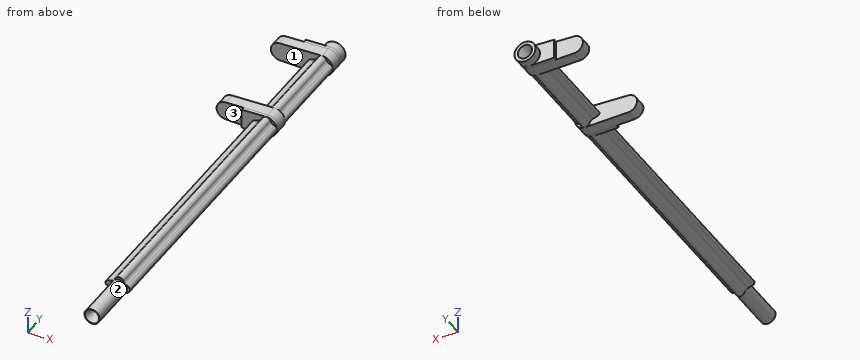
from build123d import *

# Parameters (mm, degrees)
SALIENTE_EXTRUIR2_DEPTH = 223
SALIENTE_EXTRUIR3_DEPTH = 7
SALIENTE_EXTRUIR4_DEPTH = 2
CROQUIS7_R              = 6.250085867
SALIENTE_EXTRUIR5_DEPTH = 5
CROQUIS8_R              = 4.25
CROQUIS9_R              = 1
CROQUIS10_R             = 4.57471759
SALIENTE_EXTRUIR6_DEPTH = 30


with BuildPart() as part:
    # Croquis1 → Saliente-Extruir2 (new body)
    with BuildSketch(Plane(origin=(0, 0, 0), x_dir=(1, 0, 0), z_dir=(0, 1, 0))):
        with BuildLine():
            Line((-14.479902674, 6.344412478), (-17.285197352, 5.373069954))
            ThreePointArc((-17.285197352, 5.373069954), (-18.294405629, 3.955634423), (-17.285197352, 2.538198891))
            Line((-17.285197352, 2.538198891), (-14.479902674, 1.566856368))
            ThreePointArc((-14.479902674, 1.566856368), (-13.134902489, 0.727156406), (-12.288428502, -0.61359089))
            ThreePointArc((-12.288428502, -0.61359089), (-9.893736846, -2.309516044), (-7.499045189, -0.61359089))
            ThreePointArc((-7.499045189, -0.61359089), (-6.663048477, 0.716688354), (-5.33552109, 1.557048043))
            ThreePointArc((-5.33552109, 1.557048043), (-3.642743095, 3.955634423), (-5.33552109, 6.354220802))
            ThreePointArc((-5.33552109, 6.354220802), (-6.654198374, 7.185732469), (-7.490653659, 8.501279498))
            ThreePointArc((-7.490653659, 8.501279498), (-9.893736846, 10.190483956), (-12.296820032, 8.501279498))
            ThreePointArc((-12.296820032, 8.501279498), (-13.143789356, 7.175301343), (-14.479902674, 6.344412478))
        make_face()
    extrude(amount=SALIENTE_EXTRUIR2_DEPTH)

    # Croquis5 → Saliente-Extruir3 (add)
    with BuildSketch(Plane(origin=(0, 223, 0), x_dir=(1, 0, 0), z_dir=(0, 1, 0))):
        with BuildLine():
            Line((-10.079327793, 10.188632247), (-35.332864115, 9.438053784))
            ThreePointArc((-35.332864115, 9.438053784), (-40.669466825, 3.940481472), (-35.332864115, -1.55709084))
            Line((-35.332864115, -1.55709084), (-10.079327793, -2.307669303))
            ThreePointArc((-10.079327793, -2.307669303), (-3.64271211, 3.940481472), (-10.079327793, 10.188632247))
        make_face()
    saliente_extruir3 = extrude(amount=SALIENTE_EXTRUIR3_DEPTH)

    # Croquis6 → Saliente-Extruir4 (add)
    with BuildSketch(Plane(origin=(0, 230, 0), x_dir=(1, 0, 0), z_dir=(0, 1, 0))):
        with BuildLine():
            Line((-24.6694675, 9.754988242), (-10.105220694, 10.18780896))
            ThreePointArc((-10.105220694, 10.18780896), (-3.64271211, 3.940481472), (-10.105220694, -2.306846016))
            Line((-10.105220694, -2.306846016), (-24.6694675, -1.874002597))
            Line((-24.6694675, -1.874002597), (-24.6694675, 9.754988242))
        make_face()
    saliente_extruir4 = extrude(amount=SALIENTE_EXTRUIR4_DEPTH)

    # Croquis7 → Saliente-Extruir5 (add)
    with BuildSketch(Plane(origin=(0, 232, 0), x_dir=(1, 0, 0), z_dir=(0, 1, 0))):
        with Locations((-9.919552693, 3.940481472)):
            Circle(CROQUIS7_R)
    extrude(amount=SALIENTE_EXTRUIR5_DEPTH)

    # Croquis8 → Cortar-Recubrir1 section 0
    with BuildSketch(Plane(origin=(0, 237, 0), x_dir=(1, 0, 0), z_dir=(0, 1, 0))):
        with Locations((-9.919552693, 3.940481472)):
            Circle(CROQUIS8_R)
    # Croquis9 → Cortar-Recubrir1 section 1
    with BuildSketch(Plane(origin=(0, 229, 0), x_dir=(1, 0, 0), z_dir=(0, 1, 0))):
        with Locations((-9.919552693, 3.940481472)):
            Circle(CROQUIS9_R)
    cortar_recubrir1 = loft(mode=Mode.SUBTRACT)

    # Simetría3: Saliente-Extruir3 across plane
    add(saliente_extruir3.mirror(Plane(origin=(0, 196.75, 0), x_dir=(0, 0, 1), z_dir=(0, -1, 0))))

    # Simetría4: Saliente-Extruir4 across plane
    add(saliente_extruir4.mirror(Plane(origin=(0, 196.75, 0), x_dir=(0, 0, 1), z_dir=(0, -1, 0))))

    # Croquis10 → Saliente-Extruir6 (add)
    with BuildSketch(Plane.XZ):
        with Locations((-9.893736846, -3.955634423)):
            Circle(CROQUIS10_R)
    extrude(amount=SALIENTE_EXTRUIR6_DEPTH)

    # Simetría5: Cortar-Recubrir1 across plane
    add(cortar_recubrir1.mirror(Plane(origin=(0, 103.5, 0), x_dir=(0, 0, 1), z_dir=(0, -1, 0))), mode=Mode.SUBTRACT)


solid = part.part
Can you work these out from the model? Positions are in its coordinate system, mm. Face numbers are marked on the shaded views. Coordinates: 2 decimals unless noted, no trailing zeros. Write each loop counter-clockwise with the first axis right and the second up, starting at its lowest first coordinate (ties: lowest second). Pieces come first, ordered by that corner, then holes. Notation, with made-up numbers: (28, 10.5) -> (40, 10.5) arc R20 cw to (40, 16.5) -> close; hole circle Ø9 at (58, 23). An arc over 180 degrees is marked (long way). Answer as CSV lines item,"result".
1) If we section it at C-C on x = -32: Please give me the cut outline in (y, z).
Check result:
outline,"(163.5, -9.54) -> (170.5, -9.54) -> (170.5, 1.66) -> (163.5, 1.66) -> close; (223, -9.54) -> (230, -9.54) -> (230, 1.66) -> (223, 1.66) -> close"
2) If we section it at D-D on y = -5: Please give me the cut outline in (x, z).
Check result:
outline,"circle Ø9.15 at (-9.89, -3.96)"
3) Will these pins go through, and if not, where does the flat tip stop? P1, Ø3, axis at x = -7.5, z = -4.5, coming from the +Y side; P2, Ø5, axis at x = -20, y = 209.5, coming from the +Z side; P3, Ø2, axis at x = -10.5, z = -4.5, coming from the -Y side; P4, Ø5, axis at x = -12, y = 142.5, coming from the +Z side.
Check result:
P1,"y = 236.34"
P2,"z = -2.63"
P3,"y = -23.98"
P4,"z = 2.31"
4) If we section it at B-B on y = 138: Please give me the cut outline in (x, z).
Check result:
outline,"(-17.29, -5.37) -> (-14.48, -6.34) arc R3.56 cw to (-12.3, -8.5) arc R2.55 ccw to (-7.49, -8.5) arc R3.56 cw to (-5.34, -6.35) arc R2.55 ccw to (-5.34, -1.56) arc R3.56 cw to (-7.5, 0.61) arc R2.54 ccw to (-12.29, 0.61) arc R3.56 cw to (-14.48, -1.57) -> (-17.29, -2.54) arc R1.5 ccw to start"
5) If I drill on line 1 (Y direction, x = -18, z = 0.25); line 2 (Y direction, x = -37, z = -5.5); line 3 (X direction, y = -5, z = -4.5), over which ranges is the centre line in solid material (lowest first)? Write a range as from..to.
Check result:
line 1,"161.5..170.5, 223..232"
line 2,"163.5..170.5, 223..230"
line 3,"-14.44..-5.35"
6) If we mould it in two halves opening along Y, with no side actions, what happens to the marked faces 1, 2 and 3? For each: +Y half, -Y half, draft (parallel to the pull), parting line (faces both ways), or undercut.
Check result:
face 1,"undercut"
face 2,"draft"
face 3,"-Y half"
